The model under review builds one solid part; all positions refer to its coordinate system, in mm. A direction names the side the tool comes from. Coordinates: 2 decimals unless noted, no trailing zeros. Write each loop counter-clockwise with the first axis right and the second up, starting at its lowest first coordinate (ties: lowest second). Pieces come first, ordered by that corner, then holes. Notation, with made-up numbers: (13.5, 72.5) -> (55.5, 72.5) arc R5 ccw to (55.5, 76.5) -> close; hole circle Ø5 at (66.25, -25.75). An arc over 180 degrees is marked (long way). Write each question's results on one line, items separated by ' | '.
Autodesk Inventor part; units mm, degrees
ref_plane "YZ Plane" through (0, 0, 0) normal (1, 0, 0) x (0, 1, 0)
ref_plane "XZ Plane" through (0, 0, 0) normal (0, 1, 0) x (-1, 0, 0)
ref_plane "XY Plane" through (0, 0, 0) normal (0, 0, 1) x (1, 0, 0)
sketch "Sketch1" plane through (0, 0, 0) normal (0, 1, 0) x (-1, 0, 0)
  line L0 (-14.5, 17) -> (14.5, 17)
  line L1 (14.5, 17) -> (14.5, -17)
  line L2 (14.5, -17) -> (-14.5, -17)
  line L3 (-14.5, -17) -> (-14.5, 17)
  line L4 (-14.5, 17) -> (14.5, -17) construction
  line L5 (14.5, 17) -> (-14.5, -17) construction
  circle A0 centre (-20, 17.5) radius 6
  circle A1 centre (20, 17.5) radius 6
  circle A2 centre (20, -17.5) radius 6
  circle A3 centre (-20, -17.5) radius 6
  line L6 (-16, 18.5) -> (16, 18.5)
  line L7 (16, 18.5) -> (16, -18.5)
  line L8 (16, -18.5) -> (-16, -18.5)
  line L9 (-16, -18.5) -> (-16, 18.5)
  line L10 (-16, 18.5) -> (16, -18.5) construction
  line L11 (16, 18.5) -> (-16, -18.5) construction
  point P0 (0, 0)
  point P1 (-16, -13.0279)
  point P2 (-14.0839, -18.5)
  point P3 (14.0839, -18.5)
  point P4 (16, -13.0279)
  point P5 (16, 13.0279)
  point P6 (14.0839, 18.5)
  point P7 (-14.0839, 18.5)
  point P8 (-16, 13.0279)
  point P9 (-14.5, -15.1021)
  point P10 (-14.0209, -17)
  point P11 (14.0209, -17)
  point P12 (14.5, -15.1021)
  point P13 (14.5, 15.1021)
  point P14 (14.0209, 17)
  point P15 (-14.0209, 17)
  point P16 (-14.5, 15.1021)
  dimension "d0" = 29
  dimension "d1" = 34
  dimension "d2" = 12
  dimension "d3" = 12
  dimension "d4" = 12
  dimension "d5" = 12
  dimension "d6" = 35
  dimension "d8" = 40
  dimension "d9" = 40
  dimension "d13" = 5.5
  dimension "d14" = 0.5
  dimension "d15" = 1.5
  dimension "d16" = 1.5
extrude "Extrusion1" add sketch "Sketch1" along normal blind 14 contours L3 A0 L9 L6 L0 | A0 L6 A1 L0 | L3 A3 L9 A0 | A1 L6 L7 L1 L0 | L3 L2 A3 L8 L9 | A0 L6 L9 | A1 L7 L6 | A1 L7 A2 L1 | L2 A2 L8 A3 | L9 L8 A3 | A2 L7 L8 L2 L1 | A2 L8 L7
extrude "Extrusion2" add sketch "Sketch1" along normal blind 0.2 contours L0 A1 L1 A2 L2 A3 L3 A0
hole "Hole1" at (-20, 0, -17.5) at (20, 0, -17.5) at (20, 0, 17.5) at (-20, 0, 17.5) direction (0, 1, 0) diameter 4 end through all
extrude "Extrusion3" add sketch "Sketch1" along normal blind 0.2 contours L0 A0 L3 | L0 L1 A1 | A3 L2 L3 | L1 L2 A2
sketch "Sketch2" plane through (0, 14, 0) normal (0, 1, 0) x (1, 0, 0)
  arc A0 (-16, -13.0279) -> (-14.0839, -18.5) centre (-20, -17.5) ccw
  line L0 (-17.3483, -20.5499) -> (-21.3155, -21.3214)
  line L1 (-21.3155, -21.3214) -> (-23.9671, -18.2714)
  line L2 (-23.9671, -18.2714) -> (-22.6517, -14.4501)
  line L3 (-22.6517, -14.4501) -> (-18.6845, -13.6786)
  line L4 (-18.6845, -13.6786) -> (-16.0329, -16.7286)
  line L5 (-16.0329, -16.7286) -> (-17.3483, -20.5499)
  line L6 (-10.7502, -12.1358) -> (-10.7502, 6.4156) construction
  line L7 (-10.7502, 6.4156) -> (-3.4446, 6.4156) construction
  line L8 (-22.6517, 20.5499) -> (-18.6845, 21.3214)
  line L9 (-18.6845, 21.3214) -> (-16.0329, 18.2714)
  line L10 (-16.0329, 18.2714) -> (-17.3483, 14.4501)
  line L11 (-17.3483, 14.4501) -> (-21.3155, 13.6786)
  line L12 (-21.3155, 13.6786) -> (-23.9671, 16.7286)
  line L13 (-23.9671, 16.7286) -> (-22.6517, 20.5499)
  line L14 (17.3483, -14.4501) -> (21.3155, -13.6786)
  line L15 (21.3155, -13.6786) -> (23.9671, -16.7286)
  line L16 (23.9671, -16.7286) -> (22.6517, -20.5499)
  line L17 (22.6517, -20.5499) -> (18.6845, -21.3214)
  line L18 (18.6845, -21.3214) -> (16.0329, -18.2714)
  line L19 (16.0329, -18.2714) -> (17.3483, -14.4501)
  line L20 (17.3483, 20.5499) -> (21.3155, 21.3214)
  line L21 (21.3155, 21.3214) -> (23.9671, 18.2714)
  line L22 (23.9671, 18.2714) -> (22.6517, 14.4501)
  line L23 (22.6517, 14.4501) -> (18.6845, 13.6786)
  line L24 (18.6845, 13.6786) -> (16.0329, 16.7286)
  line L25 (16.0329, 16.7286) -> (17.3483, 20.5499)
  point P0 (0, 0)
  dimension "d30" = 7
  dimension "d33" = 35
  dimension "d36" = 40
extrude "Extrusion4" cut sketch "Sketch2" against normal blind 3.2
sketch "Sketch3" plane through (-14.0839, 0, 18.5) normal (0, 0, 1) x (1, 0, 0)
  line L0 (28.1678, 14) -> (0, 14)
  arc A0 (8.0839, 14) -> (20.0839, 14) centre (14.0839, 14) ccw
  point P0 (14.0839, 0)
  dimension "d41" = 12
extrude "Extrusion5" cut sketch "Sketch3" against normal up to surface (1.5 mm away)
sketch "Sketch4" plane through (-14.5, 14, -17) normal (0, 0, 1) x (1, 0, 0)
  line L0 (0, 0) -> (29, 0)
  arc A0 (9.5, 0) -> (19.5, 0) centre (14.5, 0) ccw
  point P0 (14.5, -14)
  dimension "d44" = 10
extrude "Extrusion6" cut sketch "Sketch4" against normal through all
sketch "Sketch5" plane through (-14.0839, 0, 18.5) normal (0, 0, 1) x (1, 0, 0)
  circle A0 centre (14.0839, 4.5) radius 1.5
  line L0 (0, 0) -> (-11.9161, 0)
  point P0 (14.0839, 0)
  point P1 (-1.9161, 0)
  dimension "d47" = 3
  dimension "d48" = 4.5
extrude "Extrusion7" cut sketch "Sketch5" against normal blind 0.5
properties part number "_UCHWYT_DUZY_SILNIK"
Q1. Clearance check with flat-ended pins moving along their axes: P1, Ø4, axis at x = 6, y = 10, coming from the -Z side; P2, Ø0.9, axis at x = 0.5, y = 5, coming from the +Z side; P3, Ø2, axis at y = 5, z = -4.5, coming from the +X side. State where each tip first meets the part, or that it passes through.
Solution:
P1: z = -18.5 | P2: z = 18 | P3: x = 16
Q2. Add section A-A (y = 9.75). Write out the cut boundary in (x, z), plus the area to 3 significant figures.
Solution:
outline: (-16, -13.03) arc R6 ccw (long way) to (-14.08, -18.5) -> (-2.63, -18.5) -> (-2.63, -17) -> (-14.5, -17) -> (-14.5, 17) -> (-4.24, 17) -> (-4.24, 18.5) -> (-14.08, 18.5) arc R6 ccw (long way) to (-16, 13.03) -> close; (2.63, -18.5) -> (14.08, -18.5) arc R6 ccw (long way) to (16, -13.03) -> (16, 13.03) arc R6 ccw (long way) to (14.08, 18.5) -> (4.24, 18.5) -> (4.24, 17) -> (14.5, 17) -> (14.5, -17) -> (2.63, -17) -> close; hole circle Ø4 at (-20, -17.5); hole circle Ø4 at (-20, 17.5); hole circle Ø4 at (20, -17.5); hole circle Ø4 at (20, 17.5) | area: 547 mm²
Q3. For line 1 (X direction, y = 4, z = -17.5); line 2 (Z direction, x = 20, y = 2.5); line 3 (X direction, y = 9, z = -6.5), list the stretches that pass through material, from the lowest coordinate up. Write a range as from..to.
Solution:
line 1: -26..-22, -18..18, 22..26 | line 2: -23.5..-19.5, -15.5..-11.5, 11.5..15.5, 19.5..23.5 | line 3: -16..-14.5, 14.5..16
Q4. Add section D-D (y = 2.25). Write out the cut boundary in (x, z).
Solution:
outline: (-16, -13.03) arc R6 ccw (long way) to (-14.08, -18.5) -> (14.08, -18.5) arc R6 ccw (long way) to (16, -13.03) -> (16, 13.03) arc R6 ccw (long way) to (14.08, 18.5) -> (-14.08, 18.5) arc R6 ccw (long way) to (-16, 13.03) -> close; hole circle Ø4 at (-20, -17.5); hole circle Ø4 at (-20, 17.5); hole (-14.5, -17) -> (14.5, -17) -> (14.5, 17) -> (-14.5, 17) -> close; hole circle Ø4 at (20, -17.5); hole circle Ø4 at (20, 17.5)
Q5. Add section B-B (z = -3.5). Write out the cut boundary in (x, y), plus the area to 3 significant figures.
Solution:
outline: (-16, 0) -> (16, 0) -> (16, 14) -> (14.5, 14) -> (14.5, 0.2) -> (-14.5, 0.2) -> (-14.5, 14) -> (-16, 14) -> close | area: 47.8 mm²
Q6. Machinability: for faces 1 (the cylindrical face through (-1.5, 4.57, 18.25)), 2 (the cylindrical face through (18.017, 5.476, -17.24)), 3 (the flat face through (20.7, 12.42, 20.93)), 4 (the flat face through (0, 7, 18.5)), which of the approach directions +Z, -Z, +X, -X, +Y, -Y give a long, thin tool a straight path to every point of the face, cutting with its end or side? Answer none if there is none.
Solution:
face 1: +Z | face 2: +Y, -Y | face 3: +Y | face 4: +Z, +Y, -Y
Q7. Draft analysis for pull direction Z (two halves, no side actions). For faces 5 (the flat face through (-23.32, 12.42, -18.61)), 6 (the flat face through (0, 7, -18.5)), 7 (the cylindrical face through (0, 8, 18)), 8 (the flat face through (-22.62, 12.42, 19.82)), state which applies: pulls with the +Z half, pulls with the -Z half, needs draft (parallel to the pull), parting line crosses it, or undercut.
Solution:
face 5: undercut | face 6: pulls with the -Z half | face 7: needs draft | face 8: undercut
Q8. Add section C-C (x = 8). Write out the cut boundary in (y, z), plus the area to 3 significant figures.
Solution:
outline: (0, -18.5) -> (14, -18.5) -> (14, -17) -> (0.2, -17) -> (0.2, 17) -> (14, 17) -> (14, 18.5) -> (0, 18.5) -> close | area: 48.8 mm²
